Can you work these out from the model? Positions are in its coordinate system, mm. A direction names the side the tool comes from. Coordinates: 2 decimals unless noted, no trailing zeros. Write each loop counter-clockwise with the first axis right and the second up, starting at its lowest first coordinate (ties: lowest second). Pieces come first, ordered by that corner, then holes. Notation, with made-up numbers: (19.25, 21.25) -> (58.25, 21.25) arc R15 ccw to (58.25, 49.25) -> close; hole circle Ø8 at (-3.75, 28.25). An arc over 180 degrees is marked (long way). Answer as CSV lines item,"result". Start each with the question number.
Autodesk Inventor part; units mm, degrees
ref_plane "YZ Plane" through (0, 0, 0) normal (1, 0, 0) x (0, 1, 0)
ref_plane "XZ Plane" through (0, 0, 0) normal (0, 1, 0) x (-1, 0, 0)
ref_plane "XY Plane" through (0, 0, 0) normal (0, 0, 1) x (1, 0, 0)
sketch "Sketch1" plane through (0, 0, 0) normal (0, 1, 0) x (-1, 0, 0)
  line L0 (-100, 100) -> (100, 100)
  line L1 (100, 100) -> (100, -100)
  line L2 (100, -100) -> (-100, -100)
  line L3 (-100, -100) -> (-100, 100)
  line L4 (-100, 100) -> (100, -100) construction
  line L5 (100, 100) -> (-100, -100) construction
  point P0 (0, 0)
  dimension "d0" = 200
  dimension "d1" = 200
extrude "podstawa na mocowanie" add sketch "Sketch1" along normal blind 10
sketch "Sketch2" plane through (0, 10, 0) normal (0, 1, 0) x (1, 0, 0)
  circle A0 centre (0, 0) radius 70
  circle A1 centre (0, 0) radius 60
  dimension "d4" = 140
  dimension "d5" = 120
extrude "trzon c0" add sketch "Sketch2" along normal blind 120
sketch "Sketch5" plane through (0, 10, 0) normal (0, 1, 0) x (1, 0, 0)
  circle A0 centre (0, 0) radius 60
  circle A1 centre (0, 0) radius 60
  dimension "d19" = 120
extrude "wneka na silnik c0" cut sketch "Sketch5" against normal blind 10
sketch "Sketch6" plane through (0, 130, 0) normal (0, 1, 0) x (1, 0, 0)
  circle A0 centre (0, 0) radius 60
  dimension "d20" = 120
extrude "powierzchnia nosna dla c1" add sketch "Sketch6" against normal blind 40
sketch "Sketch8" plane through (0, 130, 0) normal (0, 1, 0) x (1, 0, 0)
  circle A0 centre (0, 0) radius 50
  dimension "d13" = 100
extrude "wneka na łożysko R0" cut sketch "Sketch8" against normal blind 18
sketch "Sketch9" plane through (0, 112, 0) normal (0, 1, 0) x (1, 0, 0)
  circle A0 centre (0, 0) radius 33
  dimension "d16" = 66
extrude "dziura na wal c1" cut sketch "Sketch9" against normal blind 22
properties part number "C0" material "Aluminum 6061"
Q1. Which directions (+Z, -Z, +X, -X, +Y, -Y) give clear straight access to the entire face, cutting with the end or side of a thin tool? Please do faces 4 (the face through (26, 90, 26)), 5 (the face through (1, 5, 100)), 6 (the face through (47.69, 121.13, -15.02)).
Q2. Imagine slicing it at C-C (y = 78.5). Write out the boundary of the cut face in (x, z), then the cut area to 3 significant figures.
Q3. Imagine slicing it at A-A (z = 0). Write out the boundary of the cut face in (x, y).
Q4. Imagine slicing it at D-D (x = 45). Write out the boundary of the cut face in (y, z), then the cut area to 3 significant figures.
Q5. I need wall thicknesses on L1, parallel to X at y = 119, z = 0; L2, parallel to X at y = 18, z = 0. Which ranges of each line are inside material? Lowest first, please.
Q6. For pin 1 (4 mm diameter, centred on y = 74.5, z = 43, fed in from +X); pin 2 (10 mm diameter, centred on x = -36, y = 100.5, fed in from +Z); pin 3 (1 mm diameter, centred on x = 47, y = 67, fed in from +Z); pin 4 (5 mm diameter, centred on x = 53, z = 23.5, fed in from -Y), each with a flat end and sliding along its axis, tell me the tip position at first contact or that it passes through.
Q7. If we mould it in two halves opening along X, with no side actions, what happens to faces 1 (the face through (-1, 5, -100)), 2 (the face through (-55.55, 69.16, -42.594)), 3 (the face through (30.5, 101.2, 12.6))? For each: released by +X, released by -X, zero draft, split by the parting line, or undercut.
Q8. Imagine slicing it at B-B (x = 0). Write out the boundary of the cut face in (y, z).
Entries:
1,face 4,"-Y"
1,face 5,"+Z, +X, -X, +Y, -Y"
1,face 6,"+Y"
2,outline,"circle Ø140 at (0, 0); hole circle Ø120 at (0, 0)"
2,area,"4,080 mm2"
3,outline,"(-100, 0) -> (-60, 0) -> (-60, 90) -> (-33, 90) -> (-33, 112) -> (-50, 112) -> (-50, 130) -> (-70, 130) -> (-70, 10) -> (-100, 10) -> close; (33, 90) -> (60, 90) -> (60, 0) -> (100, 0) -> (100, 10) -> (70, 10) -> (70, 130) -> (50, 130) -> (50, 112) -> (33, 112) -> close"
4,outline,"(0, -100) -> (10, -100) -> (10, -53.62) -> (130, -53.62) -> (130, -21.79) -> (112, -21.79) -> (112, 21.79) -> (130, 21.79) -> (130, 53.62) -> (10, 53.62) -> (10, 100) -> (0, 100) -> (0, 39.69) -> (90, 39.69) -> (90, -39.69) -> (0, -39.69) -> close"
4,area,"6,940 mm2"
5,L1,"-70 to -50, 50 to 70"
5,L2,"-70 to -60, 60 to 70"
6,pin 1,"x = 56.74"
6,pin 2,"z = 62.76"
6,pin 3,"z = 52.32"
6,pin 4,"y = 0"
7,face 1,"zero draft"
7,face 2,"split by the parting line"
7,face 3,"undercut"
8,outline,"(0, -100) -> (10, -100) -> (10, -70) -> (130, -70) -> (130, -50) -> (112, -50) -> (112, -33) -> (90, -33) -> (90, -60) -> (0, -60) -> close; (0, 60) -> (90, 60) -> (90, 33) -> (112, 33) -> (112, 50) -> (130, 50) -> (130, 70) -> (10, 70) -> (10, 100) -> (0, 100) -> close"
